Geometry check sheet. Reference: drawing and pictorial views, mm from the part's lowest x, y, z. A direction names the side the tool comes from. Give positions to 0.01 mm unless a question says otherwise; leave off trailing zeros. Write each loop counter-clockwise with the first axis right and the second up, starting at its lowest first coordinate (ties: lowest second). Pieces come first, ordered by that corner, then holes. Notation, with made-up numbers: M 7.25,-23.5 L 16.25,-23.5 A33 ccw 16.25,12.5 Z; hole C -10,24 d2. An arc over 180 degrees is marked long. Answer as a JSON object with one key per item and string values.
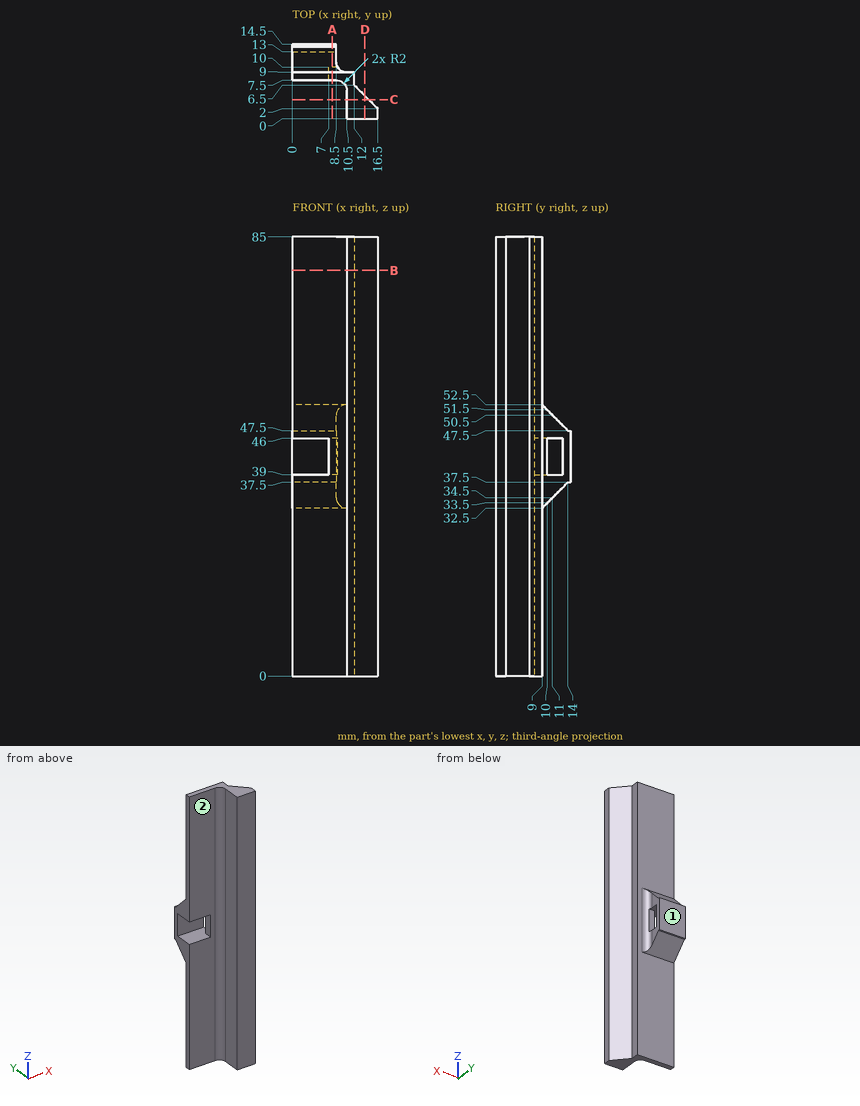
1) Section check A-A on x = 7.75. Record the boundary of the cut face in (y, z).
Completed:
{"outline": "M 7.5,0 L 9,0 L 9,32.5 L 14,37.5 L 14.5,37.5 L 14.5,47.5 L 14,47.5 L 9,52.5 L 9,85 L 7.5,85 Z; hole M 10,39 L 13,39 L 13,46 L 10,46 Z"}
2) Access from +Z, -Z, +X, -X, +Y, -Y to the whole of each face (thin tool, end or side, straight path). Record for the marked faces 1 and 2.
Completed:
{"face 1": "+Z, -Z, +X, -X, +Y", "face 2": "+Z, -Z, -X, -Y"}
3) Thickness scan on L1, parallel to X at y = 8.25, z = 9.5; L2, parallel to Z at x = 2, y = 11.25; L3, parallel to Y at x = 3.25, z = 17. Record the ranges inside material, lowest first.
Completed:
{"L1": "x = 0 to 12", "L2": "z = 34.75 to 39, 46 to 50.25", "L3": "y = 7.5 to 9"}
4) Go/stop test with flat-tipped pins: pin 1 (3 mm diameter, centred on y = 12.5, z = 43, fed in from +X); pin 2 (7.5 mm diameter, centred on x = 3.5, z = 42, fed in from -Y); pin 3 (1.3 mm diameter, centred on y = 7.5, z = 58.5, fed in from +X). Record where each tip stops, or that it passes through.
Completed:
{"pin 1": "stops at x = 8.5", "pin 2": "stops at y = 7.5", "pin 3": "stops at x = 12"}
5) Section check D-D on x = 14. Record the boundary of the cut face in (y, z).
Completed:
{"outline": "M 0,0 L 4.5,0 L 4.5,85 L 0,85 Z"}
6) Section check B-B on z = 78.5. Record the boundary of the cut face in (x, y), and give its area (3 significant figures).
Completed:
{"outline": "M 0,7.5 L 8.5,7.5 A2 cw 10.5,5.5 L 10.5,0 L 16.5,0 L 16.5,2 L 12,6.5 L 12,9 L 0,9 Z", "area": "49.2 mm2"}
7) Section check C-C on y = 3.75. Record the boundary of the cut face in (x, z).
Completed:
{"outline": "M 10.5,0 L 14.75,0 L 14.75,85 L 10.5,85 Z"}
